For this review, take the finished solid that the model builds, in its own axes (mm). Round coordinates to 2 decimals unless told otherwise and drop trailing zeros. Order: outer loops, then holes, each group sorted by start corner. A loop starts at its lowest first (then second) coordinate and runs counter-clockwise, first axis right, second up. Notation, with made-up numbers: (49.25, 79) -> (75.25, 79) arc R25 cw to (75.25, 104) -> close; hole circle Ø10 at (71.25, 15). An arc over 180 degrees is marked (long way). Answer in a Markdown table with one row per item.
Autodesk Inventor part; units mm, degrees
ref_plane "YZ Plane" through (0, 0, 0) normal (1, 0, 0) x (0, 1, 0)
ref_plane "XZ Plane" through (0, 0, 0) normal (0, 1, 0) x (-1, 0, 0)
ref_plane "XY Plane" through (0, 0, 0) normal (0, 0, 1) x (1, 0, 0)
sketch "Sketch1" plane through (0, 0, 0) normal (0, 1, 0) x (-1, 0, 0)
  line L0 (0, 0) -> (-762, 0)
  line L1 (-762, 0) -> (-762, -152.4)
  line L2 (-762, -152.4) -> (0, -152.4)
  line L3 (0, -152.4) -> (0, 0)
  line L4 (-25.4, -25.4) -> (-736.6, -25.4)
  line L5 (-736.6, -25.4) -> (-736.6, -127)
  line L6 (-736.6, -127) -> (-25.4, -127)
  line L7 (-25.4, -127) -> (-25.4, -25.4)
  line L8 (-38.1, -117.475) -> (-190.5, -117.475)
  line L9 (-190.5, -117.475) -> (-190.5, -111.125)
  line L10 (-190.5, -111.125) -> (-38.1, -111.125)
  line L11 (-38.1, -111.125) -> (-38.1, -117.475)
  line L12 (-38.1, -98.425) -> (-190.5, -98.425)
  line L13 (-190.5, -98.425) -> (-190.5, -92.075)
  line L14 (-190.5, -92.075) -> (-38.1, -92.075)
  line L15 (-38.1, -92.075) -> (-38.1, -98.425)
  line L16 (-38.1, -79.375) -> (-190.5, -79.375)
  line L17 (-190.5, -79.375) -> (-190.5, -73.025)
  line L18 (-190.5, -73.025) -> (-38.1, -73.025)
  line L19 (-38.1, -73.025) -> (-38.1, -79.375)
  line L20 (-38.1, -60.325) -> (-190.5, -60.325)
  line L21 (-190.5, -60.325) -> (-190.5, -53.975)
  line L22 (-190.5, -53.975) -> (-38.1, -53.975)
  line L23 (-38.1, -53.975) -> (-38.1, -60.325)
  line L24 (-38.1, -41.275) -> (-190.5, -41.275)
  line L25 (-190.5, -41.275) -> (-190.5, -34.925)
  line L26 (-190.5, -34.925) -> (-38.1, -34.925)
  line L27 (-38.1, -34.925) -> (-38.1, -41.275)
  line L28 (-215.9, -117.475) -> (-368.3, -117.475)
  line L29 (-368.3, -117.475) -> (-368.3, -111.125)
  line L30 (-368.3, -111.125) -> (-215.9, -111.125)
  line L31 (-215.9, -111.125) -> (-215.9, -117.475)
  line L32 (-215.9, -92.075) -> (-215.9, -98.425)
  line L33 (-215.9, -98.425) -> (-368.3, -98.425)
  line L34 (-368.3, -98.425) -> (-368.3, -92.075)
  line L35 (-368.3, -92.075) -> (-215.9, -92.075)
  line L36 (-215.9, -73.025) -> (-215.9, -79.375)
  line L37 (-215.9, -79.375) -> (-368.3, -79.375)
  line L38 (-368.3, -79.375) -> (-368.3, -73.025)
  line L39 (-368.3, -73.025) -> (-215.9, -73.025)
  line L40 (-215.9, -53.975) -> (-215.9, -60.325)
  line L41 (-215.9, -60.325) -> (-368.3, -60.325)
  line L42 (-368.3, -60.325) -> (-368.3, -53.975)
  line L43 (-368.3, -53.975) -> (-215.9, -53.975)
  line L44 (-215.9, -34.925) -> (-215.9, -41.275)
  line L45 (-215.9, -41.275) -> (-368.3, -41.275)
  line L46 (-368.3, -41.275) -> (-368.3, -34.925)
  line L47 (-368.3, -34.925) -> (-215.9, -34.925)
  line L48 (-393.7, -117.475) -> (-546.1, -117.475)
  line L49 (-546.1, -117.475) -> (-546.1, -111.125)
  line L50 (-546.1, -111.125) -> (-393.7, -111.125)
  line L51 (-393.7, -111.125) -> (-393.7, -117.475)
  line L52 (-393.7, -92.075) -> (-393.7, -98.425)
  line L53 (-393.7, -98.425) -> (-546.1, -98.425)
  line L54 (-546.1, -98.425) -> (-546.1, -92.075)
  line L55 (-546.1, -92.075) -> (-393.7, -92.075)
  line L56 (-393.7, -73.025) -> (-393.7, -79.375)
  line L57 (-393.7, -79.375) -> (-546.1, -79.375)
  line L58 (-546.1, -79.375) -> (-546.1, -73.025)
  line L59 (-546.1, -73.025) -> (-393.7, -73.025)
  line L60 (-393.7, -53.975) -> (-393.7, -60.325)
  line L61 (-393.7, -60.325) -> (-546.1, -60.325)
  line L62 (-546.1, -60.325) -> (-546.1, -53.975)
  line L63 (-546.1, -53.975) -> (-393.7, -53.975)
  line L64 (-393.7, -34.925) -> (-393.7, -41.275)
  line L65 (-393.7, -41.275) -> (-546.1, -41.275)
  line L66 (-546.1, -41.275) -> (-546.1, -34.925)
  line L67 (-546.1, -34.925) -> (-393.7, -34.925)
  line L68 (-571.5, -117.475) -> (-723.9, -117.475)
  line L69 (-723.9, -117.475) -> (-723.9, -111.125)
  line L70 (-723.9, -111.125) -> (-571.5, -111.125)
  line L71 (-571.5, -111.125) -> (-571.5, -117.475)
  line L72 (-571.5, -92.075) -> (-571.5, -98.425)
  line L73 (-571.5, -98.425) -> (-723.9, -98.425)
  line L74 (-723.9, -98.425) -> (-723.9, -92.075)
  line L75 (-723.9, -92.075) -> (-571.5, -92.075)
  line L76 (-571.5, -73.025) -> (-571.5, -79.375)
  line L77 (-571.5, -79.375) -> (-723.9, -79.375)
  line L78 (-723.9, -79.375) -> (-723.9, -73.025)
  line L79 (-723.9, -73.025) -> (-571.5, -73.025)
  line L80 (-571.5, -53.975) -> (-571.5, -60.325)
  line L81 (-571.5, -60.325) -> (-723.9, -60.325)
  line L82 (-723.9, -60.325) -> (-723.9, -53.975)
  line L83 (-723.9, -53.975) -> (-571.5, -53.975)
  line L84 (-571.5, -34.925) -> (-571.5, -41.275)
  line L85 (-571.5, -41.275) -> (-723.9, -41.275)
  line L86 (-723.9, -41.275) -> (-723.9, -34.925)
  line L87 (-723.9, -34.925) -> (-571.5, -34.925)
  dimension "d0" = 762
  dimension "d1" = 152.4
  dimension "d2" = 25.4
  dimension "d3" = 25.4
  dimension "d4" = 25.4
  dimension "d5" = 25.4
  dimension "d6" = 6.35
  dimension "d7" = 12.7
  dimension "d8" = 9.525
  dimension "d9" = 152.4
  dimension "d10" = 6.35
  dimension "d11" = 152.4
  dimension "d12" = 6.35
  dimension "d13" = 152.4
  dimension "d14" = 6.35
  dimension "d15" = 152.4
  dimension "d16" = 6.35
  dimension "d17" = 152.4
  dimension "d18" = 12.7
  dimension "d19" = 12.7
  dimension "d20" = 12.7
  dimension "d21" = 12.7
  dimension "d22" = 12.7
  dimension "d23" = 12.7
  dimension "d24" = 12.7
  dimension "d25" = 12.7
  dimension "d26" = 6.35
  dimension "d27" = 152.4
  dimension "d28" = 6.35
  dimension "d29" = 152.4
  dimension "d30" = 6.35
  dimension "d31" = 152.4
  dimension "d32" = 6.35
  dimension "d33" = 152.4
  dimension "d34" = 6.35
  dimension "d35" = 152.4
  dimension "d36" = 12.7
  dimension "d37" = 12.7
  dimension "d38" = 12.7
  dimension "d39" = 12.7
  dimension "d40" = 6.35
  dimension "d41" = 152.4
  dimension "d42" = 6.35
  dimension "d43" = 152.4
  dimension "d44" = 6.35
  dimension "d45" = 152.4
  dimension "d46" = 6.35
  dimension "d47" = 152.4
  dimension "d48" = 6.35
  dimension "d49" = 152.4
  dimension "d50" = 12.7
  dimension "d51" = 12.7
  dimension "d52" = 12.7
  dimension "d53" = 12.7
  dimension "d54" = 6.35
  dimension "d55" = 152.4
  dimension "d56" = 6.35
  dimension "d57" = 152.4
  dimension "d58" = 6.35
  dimension "d59" = 152.4
  dimension "d60" = 6.35
  dimension "d61" = 152.4
  dimension "d62" = 6.35
  dimension "d63" = 152.4
extrude "Extrusion1" add sketch "Sketch1" along normal blind 3.175 contours L3 L2 L1 L0 | L7 L6 L5 L4
properties part number "28 inch grill"
Q1. Take a section at B-B, the plane y = 0.85. Give the number of separate pieces and of enclosed holes in the cut face, then the cut area to 3 significant figures.
Answer key:
| item | result |
|---|---|
| separate pieces | 1 |
| enclosed holes | 20 |
| area | 96,800 mm^2 |
Q2. Take a section at A-A, the plane x = 293. Write out the cut boundary in (y, z) (3 decimals), then the cut area to 3 significant figures.
Answer key:
| item | result |
|---|---|
| outline | (0, -152.4) -> (3.175, -152.4) -> (3.175, -117.475) -> (0, -117.475) -> close; (0, -111.125) -> (3.175, -111.125) -> (3.175, -98.425) -> (0, -98.425) -> close; (0, -92.075) -> (3.175, -92.075) -> (3.175, -79.375) -> (0, -79.375) -> close; (0, -73.025) -> (3.175, -73.025) -> (3.175, -60.325) -> (0, -60.325) -> close; (0, -53.975) -> (3.175, -53.975) -> (3.175, -41.275) -> (0, -41.275) -> close; (0, -34.925) -> (3.175, -34.925) -> (3.175, 0) -> (0, 0) -> close |
| area | 383 mm^2 |
Q3. Clearance check with a flat-ended pin moving along its axis: pin 1 Ø1.5 at (x, y) = (471, 3) entering from +Z. State where the tip first meets the part, or that it passes through.
Answer key:
| item | result |
|---|---|
| pin 1 | stops at z = 0 |
Q4. To check wall thickness, follow probe 1 along Z at (x, y) = (65, 2.75) (3 decimals). State the ranges of the line that lie inside material, in increasing order.
Answer key:
| item | result |
|---|---|
| probe 1 | z = -152.4 to -117.475, -111.125 to -98.425, -92.075 to -79.375, -73.025 to -60.325, -53.975 to -41.275, -34.925 to 0 |
